from build123d import *

# Parameters (mm, degrees)
SKETCH_1_W             = 7
SKETCH_1_H             = 4.8
EXTRUDE_1_DEPTH        = 280
SKETCH_2_R             = 2
CUT_EXTRUDE_1_DEPTH    = 3
SKETCH_3_R             = 1
CUT_EXTRUDE_2_DEPTH    = 3
PATTERN_LINEAR_1_COUNT = 19
PATTERN_LINEAR_1_PITCH = 15
PATTERN_LINEAR_2_COUNT = 19
PATTERN_LINEAR_2_PITCH = 15


with BuildPart() as part:
    # 草图1 → 凸台-拉伸1 (new body)
    with BuildSketch(Plane.XY):
        Rectangle(SKETCH_1_W, SKETCH_1_H)
    extrude(amount=EXTRUDE_1_DEPTH)

    # 草图2 → 切除-拉伸1 (cut)
    with BuildSketch(Plane(origin=(0, 2.4, 0), x_dir=(1, 0, 0), z_dir=(0, 1, 0))):
        with Locations(Location((0, -5, 0), (0, 0, 270))):
            Circle(SKETCH_2_R)
    cut_extrude_1 = extrude(amount=-CUT_EXTRUDE_1_DEPTH, mode=Mode.SUBTRACT)

    # 草图3 → 切除-拉伸2 (cut)
    with BuildSketch(Plane(origin=(0, -0.6, 0), x_dir=(1, 0, 0), z_dir=(0, 1, 0))):
        with Locations(Location((0, -5, 0), (0, 0, 270))):
            Circle(SKETCH_3_R)
    cut_extrude_2 = extrude(amount=-CUT_EXTRUDE_2_DEPTH, mode=Mode.SUBTRACT)

    # 阵列(线性)1: 切除-拉伸2 ×19
    with Locations(*[(0, 0, i * PATTERN_LINEAR_1_PITCH) for i in range(1, PATTERN_LINEAR_1_COUNT)]):
        add(cut_extrude_2, mode=Mode.SUBTRACT)

    # 阵列(线性)2: 切除-拉伸1 ×19
    with Locations(*[(0, 0, i * PATTERN_LINEAR_2_PITCH) for i in range(1, PATTERN_LINEAR_2_COUNT)]):
        add(cut_extrude_1, mode=Mode.SUBTRACT)


solid = part.part
Verification items for the finished model (mm, model axes). Give positions to 0.01 mm unless a question says otherwise; leave off trailing zeros.
1) Depth check by flat-ended pin: pin 1 Ø3 at (x, z) = (0, 230) entering from -Y; pin 2 Ø2 at (x, z) = (-0.5, 230) entering from +Y; pin 3 Ø1.8 at (x, z) = (0, 275) entering from +Y. Enter the tip coordinate at first touch or a pass-through.
2) Thickness scan on line 1 along X through (y, z) = (1.55, 80); line 2 along Y through (x, z) = (-1.75, 95); line 3 along X through (y, z) = (-1.9, 110.5). Record the ranges inside material, lowest first.
3) Sectioned sample at A-A, the plane y = 1.45. Count the separate pieces of the cut face and the enclosed holes in it, then the cut area to 3 significant figures.
Answers:
1. pin 1: stops at y = -2.4
1. pin 2: stops at y = -0.6
1. pin 3: passes through
2. line 1: x = -3.5 to -2, 2 to 3.5
2. line 2: y = -2.4 to -0.6
2. line 3: x = -3.5 to -0.87, 0.87 to 3.5
3. separate pieces: 1
3. enclosed holes: 19
3. area: 1,720 mm2
